The listing builds one solid part. Answer for the finished solid, in the listing's coordinates (mm). A direction names the side the tool comes from. Give positions to 0.01 mm unless a question says otherwise; leave off trailing zeros. Order: outer loops, then holes, each group sorted by start corner. A loop starts at its lowest first (then second) coordinate and runs counter-clockwise, first axis right, second up. Notation, with made-up numbers: (-23.5, 82.5) - (-8.5, 82.5) arc R19 cw to (-8.5, 96.5) - close; hole circle Ø9 at (43, 17). An arc over 180 degrees is marked (long way). Answer in a Markdown table with one row per item.
from build123d import *

# Parameters (mm, degrees)
F0_W     = 60
F0_H     = 80
F1_DEPTH = 2.5
F2_W     = 4
F2_H     = 80
F3_DEPTH = 5
F3_TAPER = -20
F4_W     = 3.8198511713
F4_H     = 83.6397023427
F5_DEPTH = 5
F6_W     = 82.729776757
F6_H     = 28.9270184836
F7_DEPTH = 25


with BuildPart() as f1:
    # F0 (on Top) → F1 (new body)
    with BuildSketch(Plane.XY):
        with Locations((7.6121210307, 0.2416865528)):
            Rectangle(F0_W, F0_H)
    extrude(amount=F1_DEPTH)

    # F2 (on face) → F3 (join)
    with BuildSketch(Plane.XY.offset(2.5)):
        with Locations((-20.3878789693, 0.2416865528)):
            Rectangle(F2_W, F2_H)
    extrude(amount=F3_DEPTH, taper=F3_TAPER)

    # F4 (on face) → F5 (cut)
    with BuildSketch(Plane.XY.offset(7.5)):
        with Locations((-18.4779533836, 0.2416865528)):
            Rectangle(F4_W, F4_H)
    extrude(amount=-F5_DEPTH, mode=Mode.SUBTRACT)

    # F6 (on face) → F7 (cut)
    with BuildSketch(Plane(origin=(-18.9655101114, 0, -6.9028811582), x_dir=(0, -1, 0), z_dir=(-0.9396926208, 0, -0.3420201433))):
        with Locations((-0.6966493456, 0.8637167464)):
            Rectangle(F6_W, F6_H)
    extrude(amount=F7_DEPTH, mode=Mode.SUBTRACT)


solid = f1.part
Item 1: Each of these flat-tipped pins is pushed along its axis until it touches: P1, Ø1, axis at x = -1, y = 3.5, coming from the +Z side; P2, Ø2, axis at x = -4, z = 2, coming from the +Y side; P3, Ø3, axis at x = 4, z = 1.5, coming from the -Y side. Where does it stop, or does it pass through?
Answer block:
| item | result |
|---|---|
| P1 | z = 2.5 |
| P2 | y = 40.24 |
| P3 | y = -39.76 |
Item 2: Which of the six approach directions +Z, -Z, +X, -X, +Y, -Y give full straight-line access (tool end or side, diameter ignored) to faces 1 (the face through (-21.94, 0.8, 1.27)), 2 (the face through (-20.388, 0, 5))?
Answer block:
| item | result |
|---|---|
| face 1 | -Z, -X, +Y, -Y |
| face 2 | +Z, +X, +Y, -Y |
Item 3: Consider line 1 (Z direction, x = -16, y = 21); line 2 (Y direction, x = -2, z = 2.25); line 3 (X direction, y = 35.5, z = 2.75). Determine where each line is inside the solid, lowest interval first.
Answer block:
| item | result |
|---|---|
| line 1 | 0 to 2.5 |
| line 2 | -39.76 to 40.24 |
| line 3 | -22.48 to -20.39 |
Item 4: Find section A-A on x = 6. Write down the section's boundary in (y, z).
Answer block:
| item | result |
|---|---|
| outline | (-39.76, 0) - (40.24, 0) - (40.24, 2.5) - (-39.76, 2.5) - close |
